Model file for the job. Use its own axes, mm. A direction names the side the tool comes from. Coordinates: 2 decimals unless noted, no trailing zeros. Write each loop counter-clockwise with the first axis right and the second up, starting at its lowest first coordinate (ties: lowest second). Pieces come first, ordered by that corner, then holes.
Q1. Pull direction Y, two halves, no side cores. Call faces 1 (the flat face through (0, 15, 3)), 2 (the cylindrical face through (34, -11, 3)), 3 (the flat face through (-40, 0, 3)): released by +Y, released by -Y, zero draft, split by the parting line, or undercut.
Q2. Drill centre lines: probe 1 along Y at (x, z) = (-4, 4.7); probe 2 along Y at (x, z) = (36, 2.4); probe 3 along X at (y, z) = (11, 2.65). Where is each one in solid material? Low to high.
Q3. Band-saw the part on A-A, the plane y = -11. Write the cut outline in (x, z).
Q4. Band-saw the part on B-B, the plane x = -17. Write the cut outline in (y, z), plus the area to 3 significant figures.
Q5. Pin check, flat tip, straight feed: P1, Ø3.5, axis at x = 36, y = -11, coming from the +Z side. Stop position of the tip, or through.
Q6. Band-saw the part on C-C, the plane x = 8.5. Write the cut outline in (y, z).
Q7. Band-saw the part on D-D, the plane x = -4. Write the cut outline in (y, z).
Q8. Which spindle directions (+Z, -Z, +X, -X, +Y, -Y) get a long thin tool onto all of the face, cutting with end or side? Do faces 4 (the flat face through (32, 0, 4)), 5 (the flat face through (34, 0, 3)), 6 (the flat face through (-1, 4, 0)). Say none if no direction does.
Solid Edge part; units mm, degrees
sketch "Sketch1" plane through (0, 0, 0) normal (0, 0, 1) x (1, 0, 0)
  line L0 (-40, -15) -> (40, -15)
  line L1 (40, -15) -> (40, 15)
  line L2 (40, 15) -> (-40, 15)
  line L3 (-40, 15) -> (-40, -15)
  dimension "D1" = 40
  dimension "D2" = 40
extrude "Protrusion1" add sketch "Sketch1" along normal blind 6
sketch "Sketch2" plane through (0, 0, 6) normal (0, 0, 1) x (1, 0, 0)
  line L0 (-1, 6.25) -> (32, 6.25)
  line L1 (32, 6.25) -> (32, -6.25)
  line L2 (32, -6.25) -> (-1, -6.25)
  line L3 (-1, -6.25) -> (-1, 6.25)
  dimension "D1" = 1
  dimension "D2" = 32
extrude "Utskärning_för_batteriet" cut sketch "Sketch2" against normal blind 4
hole "Hole1" at (36, 11, 6) direction (0, 0, -1) diameter 4 end up to next
hole "Hole2" at (36, -11, 6) direction (0, 0, -1) diameter 4 end up to next
hole "Hole3" at (-4, 11, 6) direction (0, 0, -1) diameter 4 end up to next
hole "Hole4" at (-4, -11, 6) direction (0, 0, -1) diameter 4 end up to next
sketch "Sketch3" plane through (0, 0, 6) normal (0, 0, 1) x (0, -1, 0)
  line L0 (-5.2608, 38) -> (-5.2608, 34)
  line L1 (-5.2608, 34) -> (5.7392, 34)
  line L2 (5.7392, 34) -> (5.7392, 38)
  line L3 (5.7392, 38) -> (-5.2608, 38)
  line L4 (9, 31.9183) -> (9, 0.9183)
  line L5 (9, 0.9183) -> (13, 0.9183)
  line L6 (13, 0.9183) -> (13, 31.9183)
  line L7 (13, 31.9183) -> (9, 31.9183)
  line L8 (-9, 31.9183) -> (-13, 31.9183)
  line L9 (-13, 31.9183) -> (-13, 0.9183)
  line L10 (-13, 0.9183) -> (-9, 0.9183)
  line L11 (-9, 0.9183) -> (-9, 31.9183)
  line L12 (-10, -10.6932) -> (-10, -32.6932)
  line L13 (-10, -32.6932) -> (10, -32.6932)
  line L14 (10, -32.6932) -> (10, -10.6932)
  line L15 (10, -10.6932) -> (-10, -10.6932)
  dimension "D1" = 5.2608
  dimension "D2" = 5.7392
extrude "Cutout1" cut sketch "Sketch3" against normal through all
sketch "Sketch4" plane through (0, 0, 6) normal (0, 0, 1) x (0, -1, 0)
  line L0 (-2.9, -1) -> (2.9, -1)
  line L1 (2.9, -1) -> (2.9, -12.6932)
  line L2 (2.9, -12.6932) -> (-2.9, -12.6932)
  line L3 (-2.9, -12.6932) -> (-2.9, -1)
  dimension "D1" = 2.9
extrude "Cutout2" cut sketch "Sketch4" against normal through all
fillet "Avrundningar_1" radius 1 27 edges at (31.9183, -13, 3) (40, 15, 3) (32, 6.25, 4) (40, -15, 3) (0.9183, 13, 3) (32, -6.25, 4) (40, 0, 0) (0.9183, -9, 3) (34, 5.2608, 3) (38, 5.2608, 3) (31.9183, 9, 3) (0.9183, 9, 3) (-1, -6.25, 4) (-1, 6.25, 4) (31.9183, 13, 3) (38, -5.7392, 3) (-10.6932, -10, 3) (34, -5.7392, 3) (0.9183, -13, 3) (-32.6932, 10, 3) (-32.6932, -10, 3) (-10.6932, 10, 3) (-10.6932, 2.9, 3) (-10.6932, -2.9, 3) (31.9183, -9, 3) (-1, 2.9, 4) (-1, -2.9, 4)
Answer sheet:
1. face 1: released by +Y
1. face 2: undercut
1. face 3: zero draft
2. probe 1: y = -15 to -13, -9 to -2.9, 2.9 to 9, 13 to 15
2. probe 2: y = -15 to -13, -9 to -5.74, 5.26 to 9, 13 to 15
2. probe 3: x = -40 to -6, -2 to 0.92, 31.92 to 34, 38 to 40
3. outline: (-40, 0) - (-6, 0) - (-6, 6) - (-40, 6) - close; (-2, 0) - (0.92, 0) - (0.92, 6) - (-2, 6) - close; (31.92, 0) - (34, 0) - (34, 6) - (31.92, 6) - close; (38, 0) - (39, 0) arc R1 ccw to (40, 1) - (40, 6) - (38, 6) - close
4. outline: (-15, 0) - (-10, 0) - (-10, 6) - (-15, 6) - close; (10, 0) - (15, 0) - (15, 6) - (10, 6) - close
4. area: 60.0 mm2
5. P1: passes through
6. outline: (-15, 0) - (-13, 0) - (-13, 6) - (-15, 6) - close; (-9, 0) - (9, 0) - (9, 6) - (6.25, 6) - (6.25, 2) - (-6.25, 2) - (-6.25, 6) - (-9, 6) - close; (13, 0) - (15, 0) - (15, 6) - (13, 6) - close
7. outline: (-15, 0) - (-13, 0) - (-13, 6) - (-15, 6) - close; (-9, 0) - (-2.9, 0) - (-2.9, 6) - (-9, 6) - close; (2.9, 0) - (9, 0) - (9, 6) - (2.9, 6) - close; (13, 0) - (15, 0) - (15, 6) - (13, 6) - close
8. face 4: +Z
8. face 5: +Z, -Z
8. face 6: -Z, +X, -X, +Y, -Y
